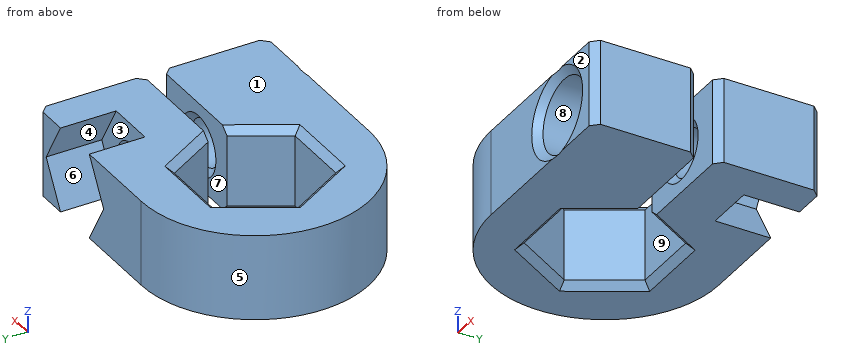
```python
from build123d import *

# Parameters (mm, degrees)
BOSS_EXTRUDE1_DEPTH = 9.525
CHAMFER1_SIZE       = 0.79375
SKETCH3_R           = 2.5527
CUT_EXTRUDE1_DEPTH  = 34.442502732
CUT_EXTRUDE2_DEPTH  = 6.2
SKETCH5_R           = 4.064
CUT_EXTRUDE3_DEPTH  = 6.35
CHAFL_N1_SIZE       = 0.79375


with BuildPart() as part:
    # Sketch2 → Boss-Extrude1 (new body)
    with BuildSketch(Plane.XY):
        with BuildLine():
            Line((3.886144662, -6.731), (7.161260289, -1.058333333))
            Line((7.161260289, -1.058333333), (9.779, -1.058333333))
            Line((9.779, -1.058333333), (19.558, -1.058333333))
            Line((19.558, -1.058333333), (19.558, -12.7))
            Line((19.558, -12.7), (0, -12.7))
            ThreePointArc((0, -12.7), (-12.7, 0), (0, 12.7))
            Line((0, 12.7), (19.558, 12.7))
            Line((19.558, 12.7), (19.558, 1.058333333))
            Line((19.558, 1.058333333), (9.779, 1.058333333))
            Line((9.779, 1.058333333), (7.161260289, 1.058333333))
            Line((7.161260289, 1.058333333), (3.886144662, 6.731))
            Line((3.886144662, 6.731), (-3.886144662, 6.731))
            Line((-3.886144662, 6.731), (-7.772289324, 0))
            Line((-7.772289324, 0), (-3.886144662, -6.731))
            Line((-3.886144662, -6.731), (3.886144662, -6.731))
        make_face()
    extrude(amount=BOSS_EXTRUDE1_DEPTH)

    # Chamfer1
    chamfer1_edges = [part.edges().sort_by_distance(p)[0] for p in [
        (5.523702475, 3.894666667, 0),
        (0, 6.731, 0),
        (-5.829216993, 3.3655, 0),
        (-5.829216993, -3.3655, 0),
        (0, -6.731, 0),
        (5.523702475, -3.894666667, 0),
        (19.558, -1.058333333, 4.7625),
        (19.558, -12.7, 4.7625),
        (19.558, 12.7, 4.7625),
        (19.558, 1.058333333, 4.7625),
        (5.523702475, -3.894666667, 9.525),
        (0, -6.731, 9.525),
        (-5.829216993, -3.3655, 9.525),
        (-5.829216993, 3.3655, 9.525),
        (0, 6.731, 9.525),
        (5.523702475, 3.894666667, 9.525),
    ]]
    chamfer(chamfer1_edges, length=CHAMFER1_SIZE)

    # Sketch3 → Cut-Extrude1 (cut, through all)
    with BuildSketch(Plane(origin=(0, 12.7, 0), x_dir=(1, 0, 0), z_dir=(0, 1, 0))):
        with Locations(Location((12.660521603, -4.7625, 0), (0, 0, 180))):
            Circle(SKETCH3_R)
    extrude(amount=-CUT_EXTRUDE1_DEPTH, mode=Mode.SUBTRACT)

    # Sketch4 → Cut-Extrude2 (cut)
    with BuildSketch(Plane(origin=(0, 12.7, 0), x_dir=(1, 0, 0), z_dir=(0, 1, 0))):
        Polygon((9.910890946, -9.525), (15.41015226, -9.525), (18.159782917, -4.7625), (15.41015226, 0), (9.910890946, 0), (7.161260289, -4.7625), align=None)
    extrude(amount=-CUT_EXTRUDE2_DEPTH, mode=Mode.SUBTRACT)

    # Sketch5 → Cut-Extrude3 (cut)
    with BuildSketch(Plane.XZ.offset(12.7)):
        with Locations((12.660521603, 4.7625)):
            Circle(SKETCH5_R)
    extrude(amount=-CUT_EXTRUDE3_DEPTH, mode=Mode.SUBTRACT)

    # Chaflán1
    # the kernel refuses this chamfer: 0.79375 mm, written as the material it takes off along each edge
    with BuildSketch(Plane(origin=(12.660521603, -1.058333333, 4.7625), x_dir=(-1, 0, 0), z_dir=(0, 0, -1))) as chafl_n1_piece_1:
        Polygon((2.5527 + CHAFL_N1_SIZE, 0), (2.5527, -CHAFL_N1_SIZE), (2.5527, 0), align=None)
    revolve(axis=Axis((12.660521603, -1.058333333, 4.7625), (0, 1, 0)), mode=Mode.SUBTRACT)
    with BuildSketch(Plane(origin=(12.660521603, 1.058333333, 4.7625), x_dir=(-1, 0, 0), z_dir=(0, 0, -1))) as chafl_n1_piece_2:
        Polygon((2.5527 + CHAFL_N1_SIZE, 0), (2.5527, CHAFL_N1_SIZE), (2.5527, 0), align=None)
    revolve(axis=Axis((12.660521603, 1.058333333, 4.7625), (0, 1, 0)), mode=Mode.SUBTRACT)
    with BuildSketch(Plane(origin=(12.660521603, -12.7, 4.7625), x_dir=(1, 0, 0), z_dir=(0, 0, -1))) as chafl_n1_piece_3:
        Polygon((4.064 + CHAFL_N1_SIZE, 0), (4.064, -CHAFL_N1_SIZE), (4.064, 0), align=None)
    revolve(axis=Axis((12.660521603, -12.7, 4.7625), (0, -1, 0)), mode=Mode.SUBTRACT)


solid = part.part
```
For this review, take the finished solid that the model builds, in its own axes (mm). Face numbers are marked on the shaded views. A direction names the side the tool comes from. Round coordinates to 2 decimals unless told otherwise and drop trailing zeros. Loops run counter-clockwise (first coordinate to the right, second up) from the corner with the lowest first, then second, coordinate; pieces in that order, holes last.
Q1. Add section A-A on x = 3.5. Write out the cut boundary in (y, z) (3 decimals), plus the area to 3 significant figures.
Result sheet:
outline: (-12.7, 0) - (-7.525, 0) - (-6.731, 0.794) - (-6.731, 8.731) - (-7.525, 9.525) - (-12.7, 9.525) - close; (6.731, 0.794) - (7.525, 0) - (12.7, 0) - (12.7, 9.525) - (7.525, 9.525) - (6.731, 8.731) - close
area: 112 mm2
Q2. Add section C-C on y = -4.25. Write out the cut boundary in (x, z) (1 decimal), plus the area to 3 significant figures.
Result sheet:
outline: (-12, 0) - (-6.2, 0) - (-5.3, 0.8) - (-5.3, 8.7) - (-6.2, 9.5) - (-12, 9.5) - close; (5.3, 0.8) - (6.2, 0) - (19.6, 0) - (19.6, 9.5) - (6.2, 9.5) - (5.3, 8.7) - close; hole circle Ø5.1 at (12.7, 4.8)
area: 177 mm2
Q3. Mouldability with a two-part tool opening along Z and no side actions: class the marked faces 1, 2, 3 and 4 as +Z half, -Z half, draft (parallel to the pull), parting line (faces both ways), or undercut.
Result sheet:
face 1: +Z half
face 2: draft
face 3: undercut
face 4: undercut
Q4. Add section B-B on y = -1.5. Write out the cut boundary in (x, z) (1 decimal), plus the area to 3 significant figures.
Result sheet:
outline: (-12.6, 0) - (-7.8, 0) - (-6.9, 0.8) - (-6.9, 8.7) - (-7.8, 9.5) - (-12.6, 9.5) - close; (6.9, 0.8) - (7.8, 0) - (19.2, 0) - (19.2, 9.5) - (7.8, 9.5) - (6.9, 8.7) - close; hole circle Ø5.8 at (12.7, 4.8)
area: 144 mm2
Q5. Insertion check: pin 1 Ø3 at (x, z) = (14.5, 5.5) entering from +Y; pin 2 Ø4 at (x, z) = (11.5, 4.5) entering from -Y; pin 3 Ø5 at (x, z) = (15.5, 2.5) entering from -Y; pin 4 Ø1 at (x, z) = (-7.5, 3) entering from -Y. Each pin has a flat end and moves straight along its axis. Give the tip position at first contact, or say it passes through.
Result sheet:
pin 1: stops at y = 6.5
pin 2: stops at y = -6.35
pin 3: stops at y = -12.7
pin 4: stops at y = -10.6
Q6. Add section D-D on x = -5.5. Write out the cut boundary in (y, z) (3 decimals).
Result sheet:
outline: (-11.447, 0) - (-5.523, 0) - (-3.936, 0.794) - (-3.936, 8.731) - (-5.523, 9.525) - (-11.447, 9.525) - close; (3.936, 0.794) - (5.523, 0) - (11.447, 0) - (11.447, 9.525) - (5.523, 9.525) - (3.936, 8.731) - close
Q7. Machinability: for the marked faces 5, 6, 7, 8 and 9, which of the approach directions +Z, -Z, +X, -X, +Y, -Y give a long, thin tool a straight path to every point of the face, cutting with its end or side? Answer none if there is none.
Result sheet:
face 5: +Z, -Z, -X
face 6: +Y
face 7: +Z, -Z, +X
face 8: -Y
face 9: +Z, -Z
Q8. To check wall thickness, follow line 1 along Y through (x, z) = (10, 7); line 2 along X through (y, z) = (4.75, 6.5); line 3 along X through (y, z) = (-1.5, 4). State the ranges of each line that lie inside material, in increasing order.
Result sheet:
line 1: y = -6.35 to -1.06, 1.06 to 6.5
line 2: x = -11.78 to -5.03, 5.03 to 10.79, 14.53 to 19.56
line 3: x = -12.61 to -6.91, 6.91 to 9.86, 15.46 to 19.21
